```python
from build123d import *

# Parameters (mm, degrees)
F1_DEPTH = 2
F1_TAPER = 45
F2_R     = 12
F2_R_2   = 10
F3_DEPTH = 5
F4_W     = 18
F4_H     = 18
F5_DEPTH = 12.5


with BuildPart() as f1:
    # F0 (on Top) → F1 (new body)
    with BuildSketch(Plane.XY):
        Polygon((-17.3205080757, -10), (0, -20), (17.3205080757, -10), (17.3205080757, 10), (0, 20), (-17.3205080757, 10), align=None)
    extrude(amount=F1_DEPTH, taper=F1_TAPER)

    # F2 (on Right) → F3 (join, symmetric)
    with BuildSketch(Plane.YZ):
        with Locations((0, 12.0482798538)):
            Circle(F2_R)
        with Locations((0, 12.0482798538)):
            Circle(F2_R_2, mode=Mode.SUBTRACT)
    extrude(amount=F3_DEPTH, both=True)

    # F4 (on Right) → F5 (cut, symmetric)
    with BuildSketch(Plane.YZ):
        with Locations((0, 22.5956004525)):
            Rectangle(F4_W, F4_H)
    extrude(amount=F5_DEPTH, both=True, mode=Mode.SUBTRACT)


solid = f1.part
```
Design review of the part built by this model. Coordinates are the model's own, in mm. A direction names the side the tool comes from. Coordinates: 2 decimals unless noted, no trailing zeros. Loops run counter-clockwise (first coordinate to the right, second up) from the corner with the lowest first, then second, coordinate; pieces in that order, holes last. Notation, with made-up numbers: (-21, 88.25) -> (19, 88.25) arc R21 cw to (19, 106.25) -> close; hole circle Ø5 at (76, 55). An arc over 180 degrees is marked (long way). Answer as a JSON object with one key per item and string values.
Q1. To check wall thickness, follow L1, parallel to Z at x = -0.5, y = 0; L2, parallel to Y at x = 1.5, z = 12; L3, parallel to X at y = 11, z = 7.5. State the ranges of each line that lie inside material, in increasing order.
Answer block:
{"L1": "z = 0 to 2.05", "L2": "y = -12 to -10, 10 to 12", "L3": "x = -5 to 5"}
Q2. Take a section at C-C on x = -3.5. Give the boundary of the cut face in (y, z), plus the area to 3 significant figures.
Answer block:
{"outline": "(-17.98, 0) -> (17.98, 0) -> (15.67, 2) -> (6.56, 2) arc R12 ccw to (9, 19.99) -> (9, 16.41) arc R10 cw (long way) to (-9, 16.41) -> (-9, 19.99) arc R12 ccw to (-6.56, 2) -> (-15.67, 2) -> close", "area": "146 mm^2"}
Q3. The part is to be moulded in two halves that separate along Y. For faces 1 (the flat face through (8.288, -14.076, 0.986)), 2 (the flat face through (0, 9, 18)), 3 (the flat face through (0, 0, 0)), say which applies: +Y half, -Y half, draft (parallel to the pull), parting line (faces both ways), or undercut.
Answer block:
{"face 1": "-Y half", "face 2": "undercut", "face 3": "draft"}
Q4. Take a section at B-B on y = 0. Give the boundary of the cut face in (x, z).
Answer block:
{"outline": "(-17.32, 0) -> (17.32, 0) -> (15.32, 2) -> (5, 2) -> (5, 2.05) -> (-5, 2.05) -> (-5, 2) -> (-15.32, 2) -> close"}
Q5. Tool access review of faces 4 (the flat face through (-5, -5, 3)), 5 (the flat face through (0, -9, 18)), 6 (the flat face through (5, -5, 3)), 7 (the cylindrical face through (-0.07, -0.283, 2.052)), 8 (the flat face through (0, -8, 2)): name each direction out of +Z, -Z, +X, -X, +Y, -Y from which nothing blocks a thin tool from reaching the whole face with its end or side.
Answer block:
{"face 4": "+Z, -X, +Y, -Y", "face 5": "+Z, +X, -X", "face 6": "+Z, +X, +Y, -Y", "face 7": "+X, -X", "face 8": "none"}
Q6. Clearance check with flat-ended pins moving along their axes: pin 1 Ø4 at (y, z) = (-3, 2.5) entering from +X; pin 2 Ø10 at (y, z) = (-9.5, 15.5) entering from +X; pin 3 Ø2 at (x, y) = (9, 15) entering from +Z. State where each tip first meets the part, or that it passes through.
Answer block:
{"pin 1": "stops at x = 16.82", "pin 2": "stops at x = 5", "pin 3": "stops at z = 0.83"}
Q7. Take a section at A-A on z = 7. Give the boundary of the cut face in (x, y).
Answer block:
{"outline": "(-5, -10.89) -> (5, -10.89) -> (5, -8.63) -> (-5, -8.63) -> close; (-5, 8.63) -> (5, 8.63) -> (5, 10.89) -> (-5, 10.89) -> close"}
Q8. Take a section at D-D on z = 4.25. Give the boundary of the cut face in (x, y).
Answer block:
{"outline": "(-5, -9.12) -> (5, -9.12) -> (5, -6.26) -> (-5, -6.26) -> close; (-5, 6.26) -> (5, 6.26) -> (5, 9.12) -> (-5, 9.12) -> close"}
